Input: dimensioned drawing with shaded views. Units: mm. Origin: part minimum x, y, z. Round coordinates to 2 decimals unless told otherwise and drop trailing zeros. Loops run counter-clockwise (first coordinate to the right, second up) from the corner with the lowest first, then second, coordinate; pieces in that order, holes last. Notation, with made-up numbers: (-0.5, 67.25) - (34.5, 67.25) arc R36 ccw to (34.5, 104.25) - close; hole circle Ø2 at (-5, 39.25). An arc over 180 degrees is marked (long way). Answer as a JSON object with one key per item and string values. Group by question number.
Item 1: Line query: line 1 (Z direction, x = 12.5, y = 17); line 2 (Z direction, x = 60, y = 18); line 3 (X direction, y = 18, z = 7). Output: solid intervals per line, ascending.
Item 2: Section B-B (x = 107.5). Return the cut outline in (y, z), plus the area to 3 significant figures.
Item 3: First-contact query: pin 1 (4 mm diameter, centred on y = 7, z = 20.5, fed in from +X); pin 2 (7 mm diameter, centred on x = 107.5, z = 30, fed in from -Y); pin 3 (6 mm diameter, centred on y = 8.5, z = 25, fed in from +X); pin 4 (6 mm diameter, centred on y = 9.5, z = 15.5, fed in from -X). Flat tips, straight axial feed; report the tip coordinate or a pass-through.
Item 4: Section D-D (z = 30). Return the cut outline in (x, y), plus the area to 3 significant figures.
Item 5: Section A-A (z = 20). Return the cut outline in (x, y).
Item 6: Section C-C (y = 17). Return the cut outline in (x, z).
Item 7: Draft query along Z for the marked faces 1, 2, 3 and 4. Return one class per face: released by +Z, released by -Z, zero draft, split by the parting line, or undercut.
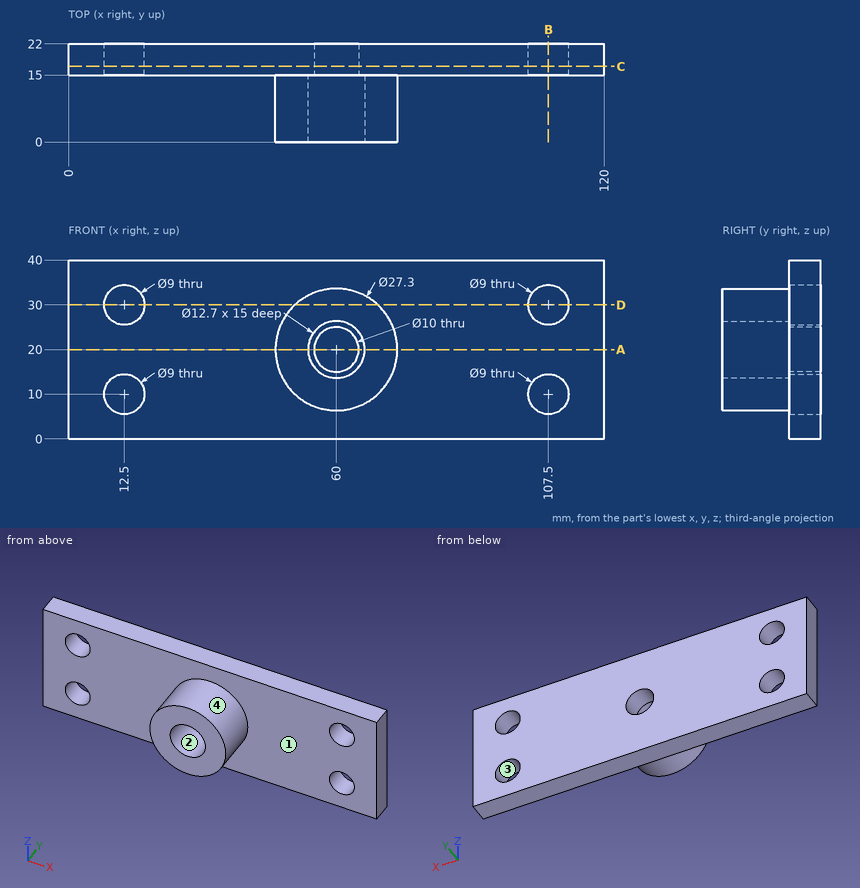
Values:
{
 "1": {"line 1": "z = 0 to 5.5, 14.5 to 25.5, 34.5 to 40", "line 2": "z = 0 to 15, 25 to 40", "line 3": "x = 0 to 9.15, 15.85 to 104.15, 110.85 to 120"},
 "2": {"outline": "(15, 0) - (22, 0) - (22, 5.5) - (15, 5.5) - close; (15, 14.5) - (22, 14.5) - (22, 25.5) - (15, 25.5) - close; (15, 34.5) - (22, 34.5) - (22, 40) - (15, 40) - close", "area": "154 mm^2"},
 "3": {"pin 1": "stops at x = 73.65", "pin 2": "passes through", "pin 3": "stops at x = 73.5", "pin 4": "stops at x = 46.43"},
 "4": {"outline": "(0, 15) - (8, 15) - (8, 22) - (0, 22) - close; (17, 15) - (50.71, 15) - (50.71, 0) - (69.29, 0) - (69.29, 15) - (103, 15) - (103, 22) - (17, 22) - close; (112, 15) - (120, 15) - (120, 22) - (112, 22) - close", "area": "993 mm^2"},
 "5": {"outline": "(0, 15) - (46.35, 15) - (46.35, 0) - (53.65, 0) - (53.65, 15) - (55, 15) - (55, 22) - (0, 22) - close; (65, 15) - (66.35, 15) - (66.35, 0) - (73.65, 0) - (73.65, 15) - (120, 15) - (120, 22) - (65, 22) - close"},
 "6": {"outline": "(0, 0) - (120, 0) - (120, 40) - (0, 40) - close; hole circle Ø9 at (12.5, 10); hole circle Ø9 at (12.5, 30); hole circle Ø10 at (60, 20); hole circle Ø9 at (107.5, 10); hole circle Ø9 at (107.5, 30)"},
 "7": {"face 1": "zero draft", "face 2": "undercut", "face 3": "undercut", "face 4": "split by the parting line"}
}
